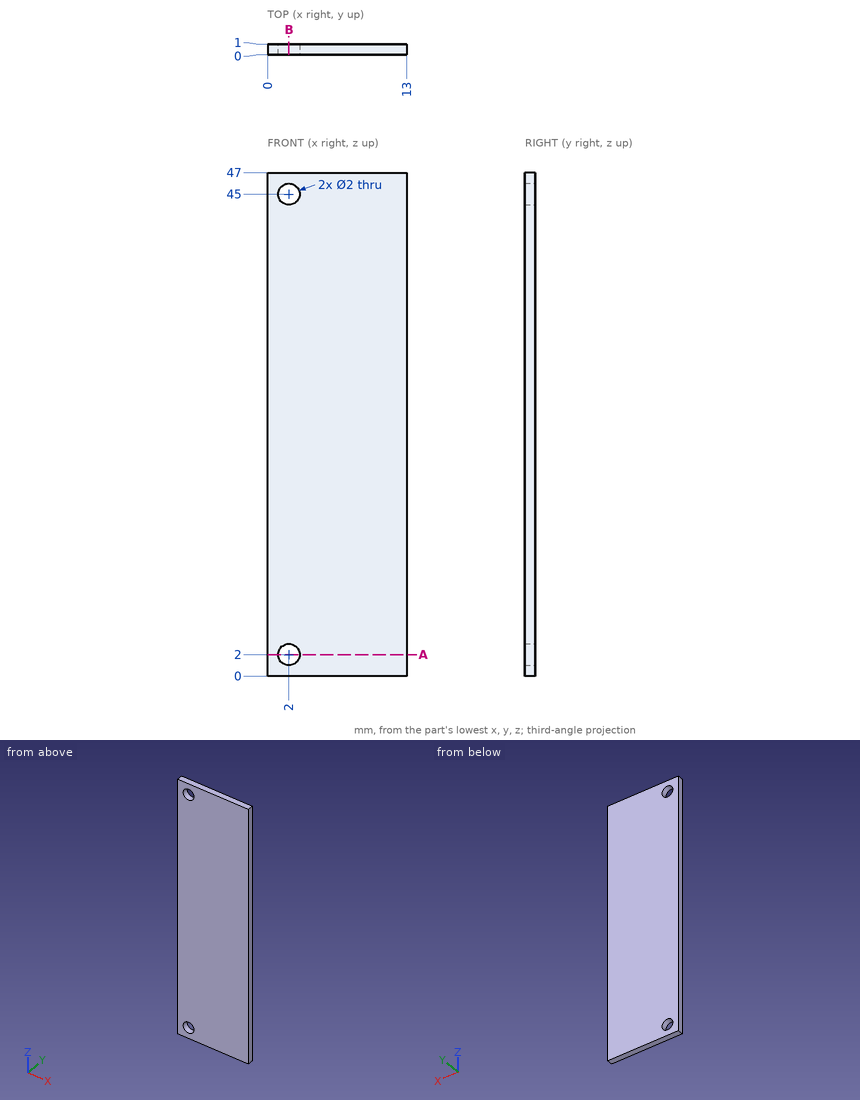
Design review of the part shown in the three views and the two pictorial views. Dimensions are in mm from the part's minimum x, y and z. Give positions to 0.01 mm unless a question says otherwise; leave off trailing zeros. Loops run counter-clockwise (first coordinate to the right, second up) from the corner with the lowest first, then second, coordinate; pieces in that order, holes last. Notation, with made-up numbers: (88.25, 16) -> (94.25, 16) arc R5 ccw to (94.25, 20) -> close; hole circle Ø6 at (16.5, 8). An arc over 180 degrees is marked (long way). Answer as a JSON object with one key per item and string values. Group by question number.
Q1. Take a section at B-B (x = 2). Write out the cut boundary in (y, z), plus the area to 3 significant figures.
Q2. Wall thickness on line 1 along Z through (x, y) = (2, 0.75); line 2 along X through (y, z) = (0.7, 2): over which ranges is each line inside the solid? List them lowest first.
Q3. Take a section at A-A (z = 2). Write out the cut boundary in (x, y), plus the area to 3 significant figures.
Answer below:
{
 "1": {"outline": "(0, 0) -> (1, 0) -> (1, 1) -> (0, 1) -> close; (0, 3) -> (1, 3) -> (1, 44) -> (0, 44) -> close; (0, 46) -> (1, 46) -> (1, 47) -> (0, 47) -> close", "area": "43.0 mm2"},
 "2": {"line 1": "z = 0 to 1, 3 to 44, 46 to 47", "line 2": "x = 0 to 1, 3 to 13"},
 "3": {"outline": "(0, 0) -> (1, 0) -> (1, 1) -> (0, 1) -> close; (3, 0) -> (13, 0) -> (13, 1) -> (3, 1) -> close", "area": "11.0 mm2"}
}
